Geometry check sheet. Reference: the model listing, model coordinates, mm. Face numbers are marked on the shaded views. Round coordinates to 2 decimals unless told otherwise and drop trailing zeros. Write each loop counter-clockwise with the first axis right and the second up, starting at its lowest first coordinate (ties: lowest second). Pieces come first, ordered by that corner, then holes.
Item 1: Draft check along Y on the marked faces 1, 2, 3 and 4. Enter one of: pulls with the +Y half, pulls with the -Y half, needs draft (parallel to the pull), parting line crosses it, or undercut.
Item 2: Cross-section at A-A (y = -14.5). Enter the section's corners in (x, z).
Item 3: Scan lines: probe 1 along X at (y, z) = (-30, 2.25); probe 2 along Y at (x, z) = (-23, 3); probe 3 along Y at (x, z) = (-10, 9.3). Record each from-to range of solid material in increasing order.
Item 4: Cross-section at B-B (x = 23). Enter the section's corners in (y, z), then the cut area to 3 significant figures.
Item 5: Cross-section at D-D (x = 10). Enter the section's corners in (y, z), then the cut area to 3 significant figures.
Item 6: Cross-section at C-C (y = 10). Enter the section's corners in (x, z).
Item 7: Depth check by flat-ended pin: P1, Ø5, axis at x = -10, y = -30, coming from the +Z side. Enter the tip coordinate at first touch or a pass-through.
from build123d import *

# Parameters (mm, degrees)
CROQUIS1_W              = 51
CROQUIS1_H              = 80
CROQUIS1_R              = 2
CROQUIS1_R_2            = 7.5
SALIENTE_EXTRUIR1_DEPTH = 12.7
CROQUIS2_R              = 4
CORTAR_EXTRUIR1_DEPTH   = 4.5


with BuildPart() as part:
    # Croquis1 → Saliente-Extruir1 (new body)
    # profile 1 of 5: a face of its own
    with BuildSketch(Plane.XY):
        with BuildLine():
            ThreePointArc((-28.5, 37), (-27.621320344, 39.121320344), (-25.5, 40))
            Line((-25.5, 40), (-30, 40))
            Line((-30, 40), (-30, -40))
            Line((-30, -40), (-28.5, -40))
            Line((-28.5, -40), (-28.5, 37))
        make_face()
    # profile 2 of 5: a face of its own
    with BuildSketch(Plane.XY):
        with BuildLine():
            Line((-25.5, -40), (-25.5, 40))
            ThreePointArc((-25.5, 40), (-27.621320344, 39.121320344), (-28.5, 37))
            Line((-28.5, 37), (-28.5, -40))
            Line((-28.5, -40), (-25.5, -40))
        make_face()
    # profile 3 of 5: a face of its own
    with BuildSketch(Plane.XY):
        Rectangle(CROQUIS1_W, CROQUIS1_H)
        with Locations((-10, -30)):
            Circle(CROQUIS1_R, mode=Mode.SUBTRACT)
        with Locations((-23, -14.5)):
            Circle(CROQUIS1_R, mode=Mode.SUBTRACT)
        with Locations((10, -30)):
            Circle(CROQUIS1_R, mode=Mode.SUBTRACT)
        with Locations((23, -14.5)):
            Circle(CROQUIS1_R, mode=Mode.SUBTRACT)
        with Locations((-23, 33)):
            Circle(CROQUIS1_R, mode=Mode.SUBTRACT)
        with Locations((0, 10)):
            Circle(CROQUIS1_R_2, mode=Mode.SUBTRACT)
        with Locations((23, 33)):
            Circle(CROQUIS1_R, mode=Mode.SUBTRACT)
    # profile 4 of 5: a face of its own
    with BuildSketch(Plane.XY):
        with BuildLine():
            ThreePointArc((28.5, 37), (27.621320344, 39.121320344), (25.5, 40))
            Line((25.5, 40), (25.5, -40))
            Line((25.5, -40), (28.5, -40))
            Line((28.5, -40), (28.5, 37))
        make_face()
    # profile 5 of 5: a face of its own
    with BuildSketch(Plane.XY):
        with BuildLine():
            Line((30, 40), (25.5, 40))
            ThreePointArc((25.5, 40), (27.621320344, 39.121320344), (28.5, 37))
            Line((28.5, 37), (28.5, -40))
            Line((28.5, -40), (30, -40))
            Line((30, -40), (30, 40))
        make_face()
    extrude(amount=SALIENTE_EXTRUIR1_DEPTH)

    # Croquis2 → Cortar-Extruir1 (cut)
    with BuildSketch(Plane.XY.offset(12.7)):
        with Locations((-10, -30)):
            Circle(CROQUIS2_R)
        with Locations((10, -30)):
            Circle(CROQUIS2_R)
    extrude(amount=-CORTAR_EXTRUIR1_DEPTH, mode=Mode.SUBTRACT)


solid = part.part
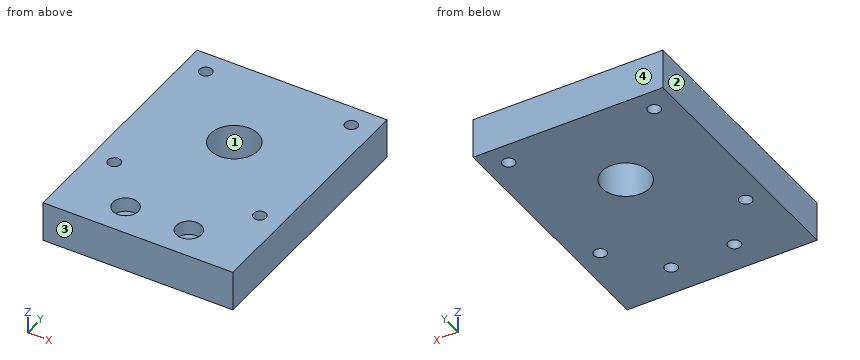
Resolved:
1. face 1: undercut
1. face 2: needs draft
1. face 3: pulls with the -Y half
1. face 4: pulls with the +Y half
2. outline: (-30, 0) - (-25, 0) - (-25, 12.7) - (-30, 12.7) - close; (-21, 0) - (21, 0) - (21, 12.7) - (-21, 12.7) - close; (25, 0) - (30, 0) - (30, 12.7) - (25, 12.7) - close
3. probe 1: x = -30 to -12, -8 to 8, 12 to 30
3. probe 2: y = -40 to -16.5, -12.5 to 31, 35 to 40
3. probe 3: y = -40 to -34, -26 to 40
4. outline: (-40, 0) - (-16.5, 0) - (-16.5, 12.7) - (-40, 12.7) - close; (-12.5, 0) - (31, 0) - (31, 12.7) - (-12.5, 12.7) - close; (35, 0) - (40, 0) - (40, 12.7) - (35, 12.7) - close
4. area: 914 mm2
5. outline: (-40, 0) - (-32, 0) - (-32, 8.2) - (-34, 8.2) - (-34, 12.7) - (-40, 12.7) - close; (-28, 0) - (40, 0) - (40, 12.7) - (-26, 12.7) - (-26, 8.2) - (-28, 8.2) - close
5. area: 947 mm2
6. outline: (-30, 0) - (-7.5, 0) - (-7.5, 12.7) - (-30, 12.7) - close; (7.5, 0) - (30, 0) - (30, 12.7) - (7.5, 12.7) - close
7. P1: stops at z = 8.2
